Can you work these out from the model? Positions are in its coordinate system, mm. Face numbers are marked on the shaded views. Give positions to 0.01 mm unless a question says otherwise; leave off trailing zeros. Order: outer loops, then holes, each group sorted by start corner. A loop starts at its lowest first (then second) coordinate and runs counter-clockwise, first axis right, second up. Notation, with made-up numbers: (84.25, -10) - (117.25, -10) arc R20 ccw to (117.25, 18) - close; hole circle Ø11 at (-22, 20). An arc over 180 degrees is marked (long way). Write each question's results on one line, items separated by ' | '. Start each with the question number.
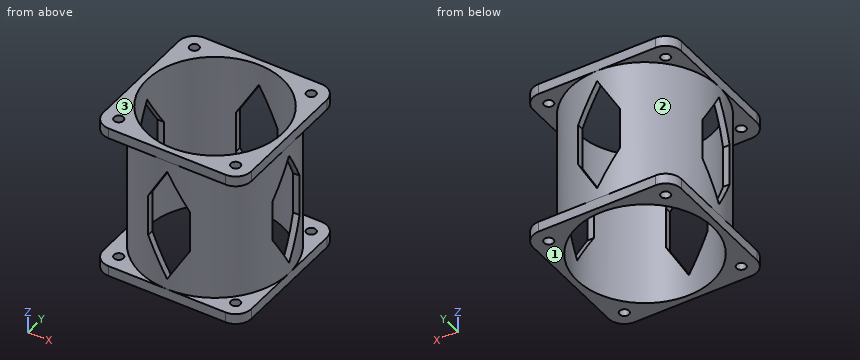
from build123d import *

# Parameters (mm, degrees)
SKETCH_R           = 35.5
SKETCH_R_2         = 32.5
PAD_DEPTH          = 75
SKETCH001_R        = 2.25
SKETCH001_R_2      = 35
PAD001_DEPTH       = 5
SKETCH002_R        = 2.25
SKETCH002_R_2      = 35
PAD002_DEPTH       = 5
POCKET_DEPTH       = 286.156142
POCKET_DEPTH_BACK  = 286.156142
POLARPATTERN_COUNT = 2
POLARPATTERN_ANGLE = 90


with BuildPart() as part:
    # Sketch → Pad (new body)
    with BuildSketch(Plane.XY):
        Circle(SKETCH_R)
        Circle(SKETCH_R_2, mode=Mode.SUBTRACT)
    extrude(amount=PAD_DEPTH)

    # Sketch001 → Pad001 (join)
    with BuildSketch(Plane.XY):
        with BuildLine():
            Line((-28, 35.5), (28, 35.5))
            ThreePointArc((35.5, 28), (33.303301, 33.303301), (28, 35.5))
            Line((35.5, 28), (35.5, -28))
            ThreePointArc((28, -35.5), (33.303301, -33.303301), (35.5, -28))
            Line((28, -35.5), (-28, -35.5))
            ThreePointArc((-35.5, -28), (-33.303301, -33.303301), (-28, -35.5))
            Line((-35.5, -28), (-35.5, 28))
            ThreePointArc((-28, 35.5), (-33.303301, 33.303301), (-35.5, 28))
        make_face()
        with Locations((-28, 28)):
            Circle(SKETCH001_R, mode=Mode.SUBTRACT)
        with Locations((28, 28)):
            Circle(SKETCH001_R, mode=Mode.SUBTRACT)
        with Locations((28, -28)):
            Circle(SKETCH001_R, mode=Mode.SUBTRACT)
        with Locations((-28, -28)):
            Circle(SKETCH001_R, mode=Mode.SUBTRACT)
        Circle(SKETCH001_R_2, mode=Mode.SUBTRACT)
    extrude(amount=PAD001_DEPTH)

    # Sketch002 → Pad002 (join)
    with BuildSketch(Plane.XY.offset(70)):
        with BuildLine():
            Line((-28, 35.5), (28, 35.5))
            ThreePointArc((35.5, 28), (33.303301, 33.303301), (28, 35.5))
            Line((35.5, 28), (35.5, -28))
            ThreePointArc((28, -35.5), (33.303301, -33.303301), (35.5, -28))
            Line((28, -35.5), (-28, -35.5))
            ThreePointArc((-35.5, -28), (-33.303301, -33.303301), (-28, -35.5))
            Line((-35.5, -28), (-35.5, 28))
            ThreePointArc((-28, 35.5), (-33.303301, 33.303301), (-35.5, 28))
        make_face()
        with Locations((-28, 28)):
            Circle(SKETCH002_R, mode=Mode.SUBTRACT)
        with Locations((28, 28)):
            Circle(SKETCH002_R, mode=Mode.SUBTRACT)
        with Locations((28, -28)):
            Circle(SKETCH002_R, mode=Mode.SUBTRACT)
        with Locations((-28, -28)):
            Circle(SKETCH002_R, mode=Mode.SUBTRACT)
        Circle(SKETCH002_R_2, mode=Mode.SUBTRACT)
    extrude(amount=PAD002_DEPTH)

    # Sketch003 → Pocket (cut, two sides)
    with BuildSketch(Plane.XZ) as pocket_sk:
        Polygon((0, 64.820508), (-10, 47.5), (-10, 27.5), (0, 10.179492), (10, 27.5), (10, 47.5), align=None)
    pocket = extrude(amount=-POCKET_DEPTH, mode=Mode.SUBTRACT) + extrude(pocket_sk.sketch, amount=POCKET_DEPTH_BACK, mode=Mode.SUBTRACT)

    # PolarPattern: Pocket ×2 about axis
    polarpattern_axis = Axis((0, 0, 0), (0, 0, 1))
    for i in range(1, POLARPATTERN_COUNT):
        add(pocket.rotate(polarpattern_axis, i * POLARPATTERN_ANGLE / (POLARPATTERN_COUNT - 1)), mode=Mode.SUBTRACT)


solid = part.part
Q1. If I drill on probe 1 along Y at (x, z) = (28, 72); probe 2 along Z at (x, y) = (-30, -26); probe 3 along X at (y, z) = (-15.5, 21), over which ranges is the centre line in solid material (lowest first)? Write a range as from..to.
Q2. Will these pins go through, and if not, where does the flat tip stop? P1, Ø6, axis at y = -7.5, z = 29.5, coming from the +X side; P2, Ø18, axis at x = -12.5, y = -20.5, coming from the -Z side; P3, Ø0.9, axis at y = 32, z = 41, coming from the +X side; P4, Ø1, axis at x = 16, z = 64.5, coming from the +Y side.
Q3. If we section it at C-C (y = 7.5): Please give me the cut outline in (x, z), plus the area to 3 significant figures.
Q4. If we section it at A-A (x = -4): Please give me the cut outline in (y, z).
Q5. If we section it at D-D (x = 19): Please give me the cut outline in (y, z).
Q6. If we section it at B-B (z = 21): Please give me the cut outline in (x, y), plus the area to 3 significant figures.
Q7. Thinking about a two-plate mould opening in Z: for the marked faces 1, 2 and 3, which applies, released by +Z, released by -Z, zero draft, split by the parting line, or undercut?
Findings below:
1) probe 1: y = -35.5..-30.25, -25.75..-16.5, 16.5..25.75, 30.25..35.5 | probe 2: z = 0..5, 70..75 | probe 3: x = -31.94..-28.57, 28.57..31.94
2) P1: stops at x = 34.06 | P2: stops at z = 0 | P3: stops at x = 16.27 | P4: stops at y = 31.94
3) outline: (-35.5, 0) - (-31.62, 0) - (-31.62, 23.17) - (-34.7, 23.17) - (-34.7, 5) - (-35.5, 5) - close; (-35.5, 70) - (-34.7, 70) - (-34.7, 51.83) - (-31.62, 51.83) - (-31.62, 75) - (-35.5, 75) - close; (31.62, 0) - (35.5, 0) - (35.5, 5) - (34.7, 5) - (34.7, 23.17) - (31.62, 23.17) - close; (31.62, 51.83) - (34.7, 51.83) - (34.7, 70) - (35.5, 70) - (35.5, 75) - (31.62, 75) - close | area: 301 mm2
4) outline: (-35.5, 0) - (-32.25, 0) - (-32.25, 17.11) - (-35.27, 17.11) - (-35.27, 5) - (-35.5, 5) - close; (-35.5, 70) - (-35.27, 70) - (-35.27, 57.89) - (-32.25, 57.89) - (-32.25, 75) - (-35.5, 75) - close; (32.25, 0) - (35.5, 0) - (35.5, 5) - (35.27, 5) - (35.27, 17.11) - (32.25, 17.11) - close; (32.25, 57.89) - (35.27, 57.89) - (35.27, 70) - (35.5, 70) - (35.5, 75) - (32.25, 75) - close
5) outline: (-35.5, 0) - (-26.37, 0) - (-26.37, 75) - (-35.5, 75) - (-35.5, 70) - (-29.99, 70) - (-29.99, 5) - (-35.5, 5) - close; (26.37, 0) - (35.5, 0) - (35.5, 5) - (29.99, 5) - (29.99, 70) - (35.5, 70) - (35.5, 75) - (26.37, 75) - close
6) outline: (-34.95, -6.25) arc R35.5 ccw to (-6.25, -34.95) - (-6.25, -31.89) arc R32.5 cw to (-31.89, -6.25) - close; (-34.95, 6.25) - (-31.89, 6.25) arc R32.5 cw to (-6.25, 31.89) - (-6.25, 34.95) arc R35.5 ccw to start; (6.25, -34.95) arc R35.5 ccw to (34.95, -6.25) - (31.89, -6.25) arc R32.5 cw to (6.25, -31.89) - close; (6.25, 31.89) arc R32.5 cw to (31.89, 6.25) - (34.95, 6.25) arc R35.5 ccw to (6.25, 34.95) - close | area: 490 mm2
7) face 1: released by -Z | face 2: undercut | face 3: released by +Z
